```python
from build123d import *

# Parameters (mm, degrees)
F1_DEPTH = 250
F3_DEPTH = 200


with BuildPart() as f1:
    # F0 (on Front) → F1 (new body, symmetric)
    with BuildSketch(Plane.XZ):
        with BuildLine():
            ThreePointArc((40, 23), (37.9497474683, 27.9497474683), (33, 30))
            Line((33, 30), (-33, 30))
            ThreePointArc((-33, 30), (-37.9497474683, 27.9497474683), (-40, 23))
            Line((-40, 23), (-40, -23))
            ThreePointArc((-40, -23), (-37.9497474683, -27.9497474683), (-33, -30))
            Line((-33, -30), (33, -30))
            ThreePointArc((33, -30), (37.9497474683, -27.9497474683), (40, -23))
            Line((40, -23), (40, 23))
        make_face()
        with BuildLine():
            Line((-33, 25), (33, 25))
            ThreePointArc((33, 25), (34.4142135624, 24.4142135624), (35, 23))
            Line((35, 23), (35, -23))
            ThreePointArc((35, -23), (34.4142135624, -24.4142135624), (33, -25))
            Line((33, -25), (-33, -25))
            ThreePointArc((-33, -25), (-34.4142135624, -24.4142135624), (-35, -23))
            Line((-35, -23), (-35, 23))
            ThreePointArc((-35, 23), (-34.4142135624, 24.4142135624), (-33, 25))
        make_face(mode=Mode.SUBTRACT)
    extrude(amount=F1_DEPTH, both=True)

    # F2 (on face) → F3 (cut)
    with BuildSketch(Plane(origin=(-40, 0, 0), x_dir=(0, -1, 0), z_dir=(-1, 0, 0))):
        Polygon((-250, -30), (-190, -30), (-197, -23), (-250, -23), align=None)
        Polygon((-250, -23), (-197, -23), (-243, 23), (-250, 23), align=None)
        Polygon((-250, 23), (-243, 23), (-250, 30), align=None)
        Polygon((243, 23), (197, -23), (250, -23), (250, 23), align=None)
        Polygon((250, -23), (197, -23), (190, -30), (250, -30), align=None)
        Polygon((250, 30), (243, 23), (250, 23), align=None)
    extrude(amount=-F3_DEPTH, mode=Mode.SUBTRACT)


solid = f1.part
```
Design review of the part built by this model. Coordinates are the model's own, in mm. A direction names the side the tool comes from. Coordinates: 2 decimals unless noted, no trailing zeros. Loops run counter-clockwise (first coordinate to the right, second up) from the corner with the lowest first, then second, coordinate; pieces in that order, holes last. Notation, with made-up numbers: (30.5, 7.25) -> (48.5, 7.25) arc R24 cw to (48.5, 24.25) -> close; hole circle Ø3 at (52.5, 25.25). An arc over 180 degrees is marked (long way). Answer as a JSON object with one key per item and string values.
Q1. Take a section at A-A on z = -0.5. Give the boundary of the cut face in (x, y).
Answer block:
{"outline": "(-40, -219.5) -> (-35, -219.5) -> (-35, 219.5) -> (-40, 219.5) -> close; (35, -219.5) -> (40, -219.5) -> (40, 219.5) -> (35, 219.5) -> close"}
Q2. To check wall thickness, follow L1, parallel to X at y = -77, z = 5.5; L2, parallel to Z at x = 6, y = 59; L3, parallel to X at y = -133, z = -23.5. State the ranges of each line that lie inside material, in increasing order.
Answer block:
{"L1": "x = -40 to -35, 35 to 40", "L2": "z = -30 to -25, 25 to 30", "L3": "x = -39.98 to -34.94, 34.94 to 39.98"}
Q3. Take a section at B-B on x = -18. Give the boundary of the cut face in (y, z).
Answer block:
{"outline": "(-250, 30) -> (-245, 25) -> (245, 25) -> (250, 30) -> close; (-195, -25) -> (-190, -30) -> (190, -30) -> (195, -25) -> close"}
Q4. Tool access review of faces 5 (the flat face through (-36, -220, 0)), 6 (the flat face through (0, -3, -25)): name each direction out of +Z, -Z, +X, -X, +Y, -Y from which nothing blocks a thin tool from reaching the whole face with its end or side.
Answer block:
{"face 5": "-Z, +X, -X, -Y", "face 6": "+Y, -Y"}
Q5. Take a section at C-C on y = 148. Give the boundary of the cut face in (x, z), plus the area to 3 significant figures.
Answer block:
{"outline": "(-40, -23) arc R7 ccw to (-33, -30) -> (33, -30) arc R7 ccw to (40, -23) -> (40, 23) arc R7 ccw to (33, 30) -> (-33, 30) arc R7 ccw to (-40, 23) -> close; hole (-35, -23) arc R2 ccw to (-33, -25) -> (33, -25) arc R2 ccw to (35, -23) -> (35, 23) arc R2 ccw to (33, 25) -> (-33, 25) arc R2 ccw to (-35, 23) -> close", "area": "1,260 mm^2"}
Q6. The part is to be moulded in two halves that separate along X. For faces 1 (the flat face through (35, -3, 0)), 2 (the flat face through (-36, 220, 0)), 3 (the flat face through (-35, -3, 0)), 4 (the flat face through (40, -3, 0)), say which applies: +X half, -X half, draft (parallel to the pull), parting line (faces both ways), or undercut.
Answer block:
{"face 1": "undercut", "face 2": "draft", "face 3": "undercut", "face 4": "+X half"}
